Answer from the drawing. Dimensions are ordinates in mm from the lowest x, y and z of the part. A direction names the side the tool comes from. Coordinates: 2 decimals unless noted, no trailing zeros. Order: outer loops, then holes, each group sorted by start corner. A loop starts at its lowest first (then second) coordinate and runs counter-clockwise, first axis right, second up.
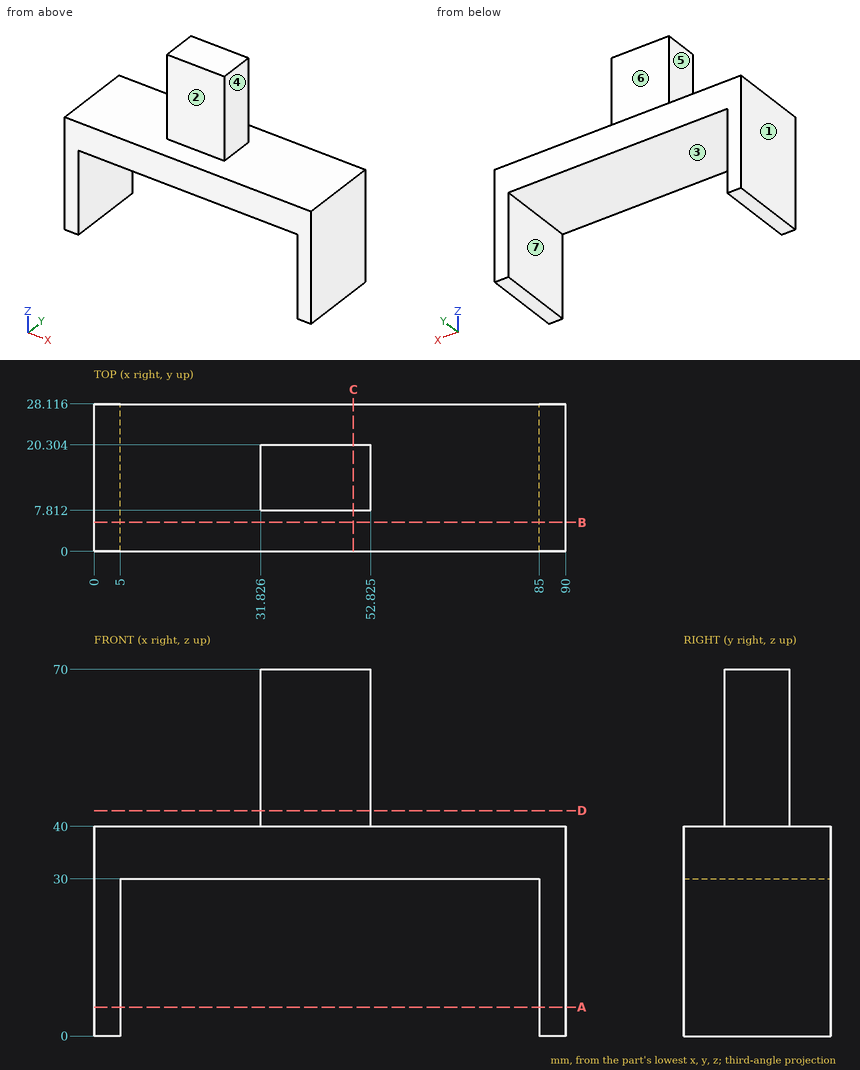
1. For the marked faces 1, 2, 3 and 4, determine the directions among +Z, -Z, +X, -X, +Y, -Y from which every point of the face is accessible in a straight line to the end or side of a thin tool.
2. The mould has two halves that part along X. Classify the marked faces 5, 6 and 7: released by +X, released by -X, zero draft, split by the parting line, or undercut.
3. The part is cut by section D-D (z = 43). Determine the outline of the cut face in (x, y) (1 decimal), plus the area to 3 significant figures.
4. The part is cut by section B-B (y = 5.5). Determine the outline of the cut face in (x, z), plus the area to 3 significant figures.
5. The part is cut by section A-A (z = 5.5). Determine the outline of the cut face in (x, y) (1 decimal), plus the area to 3 significant figures.
6. Flat-ended cylindrical pins translate along their axes: pin 1 (13.5 mm diameter, centred on y = 16, z = 58, fed in from -X); pin 2 (1 mm diameter, centred on x = 33, y = 19, fed in from -Z); pin 3 (3 mm diameter, centred on y = 10, z = 45, fed in from +X) (3 decimals); pin 4 (3 mm diameter, centred on x = 71, z = 42.5, fed in from +Y). Find the tip coordinate at first contact, or state that the pin passes through.
7. Consider probe 1 along X at (y, z) = (14, 18); probe 2 along Z at (x, y) = (64.5, 15); probe 3 along X at (y, z) = (17.25, 48.5) (1 decimal). Determine where each line is inside the solid, lowest interval first.
8. The part is cut by section C-C (x = 49.5). Determine the outline of the cut face in (y, z) (1 decimal).
Worked out:
1. face 1: +Z, -Z, -X, +Y, -Y
1. face 2: +Z, +X, -X, -Y
1. face 3: -Z, +Y, -Y
1. face 4: +Z, +X, +Y, -Y
2. face 5: released by -X
2. face 6: zero draft
2. face 7: undercut
3. outline: (31.8, 7.8) - (52.8, 7.8) - (52.8, 20.3) - (31.8, 20.3) - close
3. area: 262 mm2
4. outline: (0, 0) - (5, 0) - (5, 30) - (85, 30) - (85, 0) - (90, 0) - (90, 40) - (0, 40) - close
4. area: 1,200 mm2
5. outline: (0, 0) - (5, 0) - (5, 28.1) - (0, 28.1) - close; (85, 0) - (90, 0) - (90, 28.1) - (85, 28.1) - close
5. area: 281 mm2
6. pin 1: stops at x = 31.83
6. pin 2: stops at z = 30
6. pin 3: stops at x = 52.825
6. pin 4: passes through
7. probe 1: x = 0 to 5, 85 to 90
7. probe 2: z = 30 to 40
7. probe 3: x = 31.8 to 52.8
8. outline: (0, 30) - (28.1, 30) - (28.1, 40) - (20.3, 40) - (20.3, 70) - (7.8, 70) - (7.8, 40) - (0, 40) - close
